from build123d import *

# Parameters (mm, degrees)
SKETCH_1_R      = 1.6
EXTRUDE_1_DEPTH = 3
FILLET_1_R      = 3
FILLET_2_R      = 15


with BuildPart() as part:
    # 草图1 → 凸台-拉伸1 (new body)
    with BuildSketch(Plane.XY):
        Polygon((0, 0), (60, 0), (60, -20), (40, -40), (20, -40), (20, -20), (0, -20), align=None)
        with Locations((5, -5)):
            Circle(SKETCH_1_R, mode=Mode.SUBTRACT)
        with Locations(Location((15, -5, 0), (0, 0, 180))):
            Circle(SKETCH_1_R, mode=Mode.SUBTRACT)
        with Locations((15, -15)):
            Circle(SKETCH_1_R, mode=Mode.SUBTRACT)
        with Locations(Location((5, -15, 0), (0, 0, 180))):
            Circle(SKETCH_1_R, mode=Mode.SUBTRACT)
        with Locations((55, -15)):
            Circle(SKETCH_1_R, mode=Mode.SUBTRACT)
        with Locations(Location((45, -15, 0), (0, 0, 180))):
            Circle(SKETCH_1_R, mode=Mode.SUBTRACT)
        with Locations((45, -5)):
            Circle(SKETCH_1_R, mode=Mode.SUBTRACT)
        with Locations(Location((55, -5, 0), (0, 0, 180))):
            Circle(SKETCH_1_R, mode=Mode.SUBTRACT)
        with Locations((25, -35)):
            Circle(SKETCH_1_R, mode=Mode.SUBTRACT)
        with Locations(Location((35, -35, 0), (0, 0, 180))):
            Circle(SKETCH_1_R, mode=Mode.SUBTRACT)
        with Locations((35, -25)):
            Circle(SKETCH_1_R, mode=Mode.SUBTRACT)
        with Locations(Location((25, -25, 0), (0, 0, 180))):
            Circle(SKETCH_1_R, mode=Mode.SUBTRACT)
        Polygon((23, -5), (23, -15), (33, -15), align=None, mode=Mode.SUBTRACT)
        Polygon((27, -5), (37, -5), (37, -15), align=None, mode=Mode.SUBTRACT)
    extrude(amount=EXTRUDE_1_DEPTH)

    # 圆角1
    fillet_1_edges = [part.edges().sort_by_distance(p)[0] for p in [
        (0, 0, 1.5),
        (60, 0, 1.5),
        (60, -20, 1.5),
        (40, -40, 1.5),
        (20, -40, 1.5),
        (0, -20, 1.5),
    ]]
    fillet(fillet_1_edges, radius=FILLET_1_R)

    # 圆角2
    fillet_2_edges = [part.edges().sort_by_distance(p)[0] for p in [
        (20, -20, 1.5),
    ]]
    fillet(fillet_2_edges, radius=FILLET_2_R)


solid = part.part
Part model, mm, in its own coordinate system. A direction names the side the tool comes from. Coordinates: 2 decimals unless noted, no trailing zeros. Order: outer loops, then holes, each group sorted by start corner. A loop starts at its lowest first (then second) coordinate and runs counter-clockwise, first axis right, second up.
(1) Slice it at A-A, the plane y = -7.5. Write the cut outline in (x, z).
Check sheet entries:
outline: (0, 0) - (23, 0) - (23, 3) - (0, 3) - close; (25.5, 0) - (29.5, 0) - (29.5, 3) - (25.5, 3) - close; (37, 0) - (60, 0) - (60, 3) - (37, 3) - close
(2) Slice it at B-B, the plane x = 45. Write the cut outline in (y, z), and give its area (3 significant figures).
Check sheet entries:
outline: (-35, 0) - (-16.6, 0) - (-16.6, 3) - (-35, 3) - close; (-13.4, 0) - (-6.6, 0) - (-6.6, 3) - (-13.4, 3) - close; (-3.4, 0) - (0, 0) - (0, 3) - (-3.4, 3) - close
area: 85.8 mm2
(3) Pull direction Y, two halves, no side cores. Call faces 1 (the face through (0.9, -0.86, 1.52)), 2 (the face through (43.82, -3.92, 1.48)), 3 (the face through (50, -30, 1)): pulls with the +Y half, pulls with the -Y half, needs draft (parallel to the pull), parting line crosses it, or undercut.
Check sheet entries:
face 1: pulls with the +Y half
face 2: undercut
face 3: pulls with the -Y half
(4) Tool access for faces 4 (the face through (20.86, -39.1, 1.52)), 5 (the face through (32, -10, 1)): list every direction of +Z, -Z, +X, -X, +Y, -Y with a clear straight run to the whole face (end or side of a thin tool).
Check sheet entries:
face 4: +Z, -Z, -X, -Y
face 5: +Z, -Z
(5) Slice it at C-C, the plane x = 25. Write the cut outline in (y, z).
Check sheet entries:
outline: (-40, 0) - (-36.6, 0) - (-36.6, 3) - (-40, 3) - close; (-33.4, 0) - (-26.6, 0) - (-26.6, 3) - (-33.4, 3) - close; (-23.4, 0) - (-15, 0) - (-15, 3) - (-23.4, 3) - close; (-7, 0) - (0, 0) - (0, 3) - (-7, 3) - close
(6) Slice it at D-D, the plane z = 1.7. State how many separate pieces and enclosed holes the cut face has, and give its area (3 significant figures).
Check sheet entries:
separate pieces: 1
enclosed holes: 14
area: 1,640 mm2
(7) Probe L1, parallel to Y at x = 56, z = 2.5; L2, parallel to Y at x = 55, z = 1.4; L3, parallel to X at y = -34, z = 2.7. List the from-to ranges inside material, lowest first.
Check sheet entries:
L1: y = -24 to -16.25, -13.75 to -6.25, -3.75 to 0
L2: y = -25 to -16.6, -13.4 to -6.6, -3.4 to 0
L3: x = 19.97 to 23.75, 26.25 to 33.75, 36.25 to 46
(8) Pin check, flat tips, straight feed: pin 1 Ø1.9 at (x, y) = (25, -35) entering from +Z; pin 2 Ø1 at (y, z) = (-32, 0.5) entering from -X; pin 3 Ø1.5 at (x, z) = (15.5, 2.5) entering from -Y; pin 4 Ø1 at (x, z) = (4, 2) entering from -Y. Stop position of each tip, or through.
Check sheet entries:
pin 1: passes through
pin 2: stops at x = 19.59
pin 3: stops at y = -25.08
pin 4: stops at y = -20
